Here's how the part is built. I have some questions about the finished solid (model axes, mm). A direction names the side the tool comes from. Round coordinates to 2 decimals unless told otherwise and drop trailing zeros. Loops run counter-clockwise (first coordinate to the right, second up) from the corner with the lowest first, then second, coordinate; pieces in that order, holes last. Notation, with made-up numbers: M 8,47.25 L 37,47.25 A25 ccw 37,66.25 Z; hole C -9,62 d10. An arc over 180 degrees is marked long. Use a Markdown table: item, result.
from build123d import *

# Parameters (mm, degrees)
F0_W     = 25.4
F0_H     = 50.8
F0_W_2   = 22.225
F0_H_2   = 47.625
F1_DEPTH = 304.8
F2_R     = 7.9375
F3_DEPTH = 1.5875
F4_R     = 0.889
F5_DEPTH = 1.5875


with BuildPart() as f1:
    # F0 (on Front) → F1 (new body)
    with BuildSketch(Plane.XZ):
        Rectangle(F0_W, F0_H)
        Rectangle(F0_W_2, F0_H_2, mode=Mode.SUBTRACT)
    extrude(amount=F1_DEPTH)

    # F2 (on face) → F3 (cut)
    with BuildSketch(Plane(origin=(-12.7, 0, 0), x_dir=(0, -1, 0), z_dir=(-1, 0, 0))):
        with Locations((152.4, 0)):
            Circle(F2_R)
    extrude(amount=-F3_DEPTH, mode=Mode.SUBTRACT)

    # F4 (on face) → F5 (cut)
    with BuildSketch(Plane.YZ.offset(12.7)):
        with Locations((-152.4, 0)):
            Circle(F4_R)
    extrude(amount=-F5_DEPTH, mode=Mode.SUBTRACT)


solid = f1.part
1. Imagine slicing it at A-A, the plane z = -11. Write out the boundary of the cut face in (x, y), then the cut area to 3 significant figures.
Answer sheet:
| item | result |
|---|---|
| outline | M -12.7,-304.8 L -11.11,-304.8 L -11.11,0 L -12.7,0 Z; M 11.11,-304.8 L 12.7,-304.8 L 12.7,0 L 11.11,0 Z |
| area | 968 mm2 |
2. Which directions (+Z, -Z, +X, -X, +Y, -Y) give clear straight access to the entire face, cutting with the end or side of a thin tool? Please do faces 1 (the face through (0, -150, 23.812)), 2 (the face through (-11.917, -159.971, 2.384)), 3 (the face through (-11.3, -304.8, 2)).
Answer sheet:
| item | result |
|---|---|
| face 1 | +Y, -Y |
| face 2 | -X |
| face 3 | +Z, -Z, +X, -X, -Y |
3. Imagine slicing it at B-B, the plane y = -189.5. Write out the boundary of the cut face in (x, z).
Answer sheet:
| item | result |
|---|---|
| outline | M -12.7,-25.4 L 12.7,-25.4 L 12.7,25.4 L -12.7,25.4 Z; hole M -11.11,-23.81 L 11.11,-23.81 L 11.11,23.81 L -11.11,23.81 Z |
4. We'd pull the mould along X, two halves only. Please class faces 4 (the face through (11.112, -150, 0)), 5 (the face through (0, -150, -25.4)), 6 (the face through (-12.7, -150, 11)): +X half, -X half, draft (parallel to the pull), parting line (faces both ways), or undercut.
Answer sheet:
| item | result |
|---|---|
| face 4 | undercut |
| face 5 | draft |
| face 6 | -X half |
5. Imagine slicing it at C-C, the plane x = -7.25. Write out the boundary of the cut face in (y, z), then the cut area to 3 significant figures.
Answer sheet:
| item | result |
|---|---|
| outline | M -304.8,-25.4 L 0,-25.4 L 0,-23.81 L -304.8,-23.81 Z; M -304.8,23.81 L 0,23.81 L 0,25.4 L -304.8,25.4 Z |
| area | 968 mm2 |
6. I need wall thicknesses on probe 1 along Z at (x, y) = (12.25, -152.4); probe 2 along Z at (x, y) = (-11.65, -152.4); probe 3 along X at (y, z) = (-160, -8.5). Which ranges of each line are inside material? Lowest first, please. Write a range as from..to.
Answer sheet:
| item | result |
|---|---|
| probe 1 | -25.4..-0.89, 0.89..25.4 |
| probe 2 | -25.4..-7.94, 7.94..25.4 |
| probe 3 | -12.7..-11.11, 11.11..12.7 |
